Build history of the part. All positions in model axes, mm. Face numbers are marked on the shaded views. A direction names the side the tool comes from. Coordinates: 2 decimals unless noted, no trailing zeros. Order: outer loops, then holes, each group sorted by start corner. A loop starts at its lowest first (then second) coordinate and runs counter-clockwise, first axis right, second up. Notation, with made-up numbers: (74, 10.5) -> (83, 10.5) arc R32 ccw to (83, 49.5) -> close; hole circle Ø11 at (9.5, 58). An arc over 180 degrees is marked (long way). Write each question's results on one line, items separated by ' | '.
from build123d import *

# Parameters (mm, degrees)
SKETCH1_W           = 18.5
SKETCH1_H           = 16.5
SKETCH1_W_2         = 12.5
SKETCH1_H_2         = 10.5
BOSS_EXTRUDE1_DEPTH = 3
FILLET1_R           = 4


with BuildPart() as part:
    # Sketch1 → Boss-Extrude1 (new body)
    with BuildSketch(Plane.XY):
        Rectangle(SKETCH1_W, SKETCH1_H)
        Rectangle(SKETCH1_W_2, SKETCH1_H_2, mode=Mode.SUBTRACT)
    extrude(amount=BOSS_EXTRUDE1_DEPTH)

    # Fillet1
    fillet1_edges = [part.edges().sort_by_distance(p)[0] for p in [
        (6.25, -5.25, 1.5),
        (6.25, 5.25, 1.5),
        (-6.25, 5.25, 1.5),
        (-6.25, -5.25, 1.5),
        (9.25, -8.25, 1.5),
        (-9.25, -8.25, 1.5),
        (-9.25, 8.25, 1.5),
        (9.25, 8.25, 1.5),
    ]]
    fillet(fillet1_edges, radius=FILLET1_R)


solid = part.part
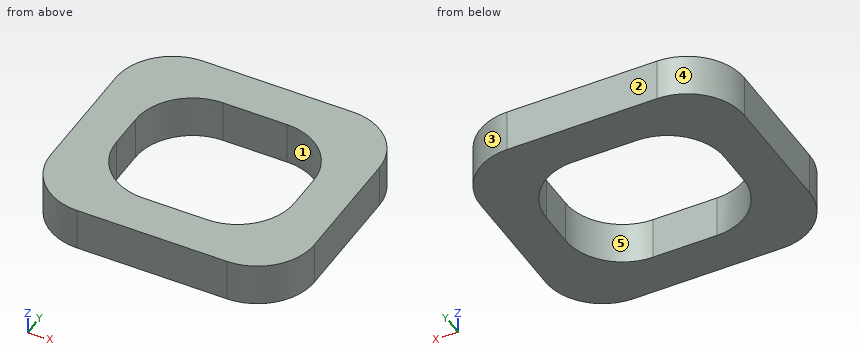
Item 1: Slice it at A-A, the plane z = 0.4. List the corners of the cut face in (x, y), and give its area (3 significant figures).
Answer:
outline: (-9.25, -4.25) arc R4 ccw to (-5.25, -8.25) -> (5.25, -8.25) arc R4 ccw to (9.25, -4.25) -> (9.25, 4.25) arc R4 ccw to (5.25, 8.25) -> (-5.25, 8.25) arc R4 ccw to (-9.25, 4.25) -> close; hole (-6.25, -1.25) arc R4 ccw to (-2.25, -5.25) -> (2.25, -5.25) arc R4 ccw to (6.25, -1.25) -> (6.25, 1.25) arc R4 ccw to (2.25, 5.25) -> (-2.25, 5.25) arc R4 ccw to (-6.25, 1.25) -> close | area: 174 mm^2
Item 2: Drill centre lines: line 1 (Y direction, x = 0, z = 0.6); line 2 (X direction, y = 0, z = 2.05); line 3 (Y direction, x = 4.5, z = 0.95). Where is each one in solid material? Low to high. Write a range as from..to.
Answer:
line 1: y = -8.25..-5.25, 5.25..8.25 | line 2: x = -9.25..-6.25, 6.25..9.25 | line 3: y = -8.25..-4.56, 4.56..8.25
Item 3: Slice it at D-D, the plane y = 5.75. List the corners of the cut face in (x, z), and give its area (3 significant figures).
Answer:
outline: (-8.96, 0) -> (8.96, 0) -> (8.96, 3) -> (-8.96, 3) -> close | area: 53.7 mm^2
Item 4: Tool access for the marked faces 1 and 2: list every direction of +Z, -Z, +X, -X, +Y, -Y with a clear straight run to the whole face (end or side of a thin tool).
Answer:
face 1: +Z, -Z | face 2: +Z, -Z, +X, -X, +Y
Item 5: Slice it at C-C, the plane x = -1.25. List the corners of the cut face in (y, z), and give its area (3 significant figures).
Answer:
outline: (-8.25, 0) -> (-5.25, 0) -> (-5.25, 3) -> (-8.25, 3) -> close; (5.25, 0) -> (8.25, 0) -> (8.25, 3) -> (5.25, 3) -> close | area: 18.0 mm^2
Item 6: Slice it at B-B, the plane y = 0.75. List the corners of the cut face in (x, z), and give its area (3 significant figures).
Answer:
outline: (-9.25, 0) -> (-6.25, 0) -> (-6.25, 3) -> (-9.25, 3) -> close; (6.25, 0) -> (9.25, 0) -> (9.25, 3) -> (6.25, 3) -> close | area: 18.0 mm^2
Item 7: Pin check, flat tip, straight feed: pin 1 (1.5 mm diameter, centred on x = 5, y = 2, fed in from +Z). Stop position of the tip, or through.
Answer:
pin 1: passes through
Item 8: Pull direction X, two halves, no side cores. Call the marked faces 3, 4 and 5: released by +X, released by -X, zero draft, split by the parting line, or undercut.
Answer:
face 3: released by +X | face 4: released by -X | face 5: undercut
